from build123d import *

# Parameters (mm, degrees)
CROQUIS1_R              = 2.5
CROQUIS1_R_2            = 37.5
CROQUIS1_R_3            = 15
CROQUIS1_R_4            = 2.25
CROQUIS1_R_5            = 1.5
CROQUIS1_W              = 150
CROQUIS1_H              = 150
SALIENTE_EXTRUIR1_DEPTH = 10


with BuildPart() as part:
    # Croquis1 → Saliente-Extruir1 (new body)
    with BuildSketch(Plane.XY):
        with BuildLine():
            Line((15, 0), (485, 0))
            ThreePointArc((485, 0), (495.606601718, 4.393398282), (500, 15))
            Line((500, 15), (500, 235))
            ThreePointArc((500, 235), (495.606601718, 245.606601718), (485, 250))
            Line((485, 250), (15, 250))
            ThreePointArc((15, 250), (4.393398282, 245.606601718), (0, 235))
            Line((0, 235), (0, 15))
            ThreePointArc((0, 15), (4.393398282, 4.393398282), (15, 0))
        make_face()
        with Locations((110, 185.621778265)):
            Circle(CROQUIS1_R, mode=Mode.SUBTRACT)
        with Locations((162.5, 94.689110868)):
            Circle(CROQUIS1_R, mode=Mode.SUBTRACT)
        with Locations((57.5, 94.689110868)):
            Circle(CROQUIS1_R, mode=Mode.SUBTRACT)
        with Locations((110, 125)):
            Circle(CROQUIS1_R_2, mode=Mode.SUBTRACT)
        with Locations((230, 235)):
            Circle(CROQUIS1_R, mode=Mode.SUBTRACT)
        with Locations((270, 235)):
            Circle(CROQUIS1_R, mode=Mode.SUBTRACT)
        with Locations((189.096460098, 45)):
            Circle(CROQUIS1_R_3, mode=Mode.SUBTRACT)
        with Locations((475, 210)):
            Circle(CROQUIS1_R_4, mode=Mode.SUBTRACT)
        with Locations((305, 210)):
            Circle(CROQUIS1_R_4, mode=Mode.SUBTRACT)
        with Locations((305, 40)):
            Circle(CROQUIS1_R_4, mode=Mode.SUBTRACT)
        with Locations((475, 40)):
            Circle(CROQUIS1_R_4, mode=Mode.SUBTRACT)
        with Locations((350, 10)):
            Circle(CROQUIS1_R, mode=Mode.SUBTRACT)
        with Locations((380, 10)):
            Circle(CROQUIS1_R, mode=Mode.SUBTRACT)
        with Locations(Location((120, 10, 0), (0, 0, 180))):
            Circle(CROQUIS1_R, mode=Mode.SUBTRACT)
        with Locations(Location((150, 10, 0), (0, 0, 180))):
            Circle(CROQUIS1_R, mode=Mode.SUBTRACT)
        with Locations((240, 125)):
            Circle(CROQUIS1_R, mode=Mode.SUBTRACT)
        with Locations((260, 125)):
            Circle(CROQUIS1_R, mode=Mode.SUBTRACT)
        with Locations((250, 125)):
            Circle(CROQUIS1_R_5, mode=Mode.SUBTRACT)
        with Locations((390, 125)):
            Rectangle(CROQUIS1_W, CROQUIS1_H, mode=Mode.SUBTRACT)
    extrude(amount=SALIENTE_EXTRUIR1_DEPTH)


solid = part.part
Geometry: final body of the model. Coordinates: model frame, mm. A direction names the side the tool comes from. Round coordinates to 2 decimals unless told otherwise and drop trailing zeros. Order: outer loops, then holes, each group sorted by start corner. A loop starts at its lowest first (then second) coordinate and runs counter-clockwise, first axis right, second up. Notation, with made-up numbers: (79, -1) -> (84, -1) arc R14 cw to (84, 26) -> close; hole circle Ø11 at (7.25, 52.25). An arc over 180 degrees is marked (long way). Put each result on its own line as item: value. Start each with the question number.
Q1. Section C-C on y = 148. Return the cut outline in (x, z), and give its area (3 significant figures).
Q2. Line query: probe 1 along Y at (x, z) = (110, 3); probe 2 along X at (y, z) = (235, 6); probe 3 along Y at (x, z) = (305, 2). Output: solid intervals per line, ascending.
Q3. First-contact query: pin 1 (3 mm diameter, centred on x = 240, y = 125, fed in from +Z). Flat tip, straight axial feed; report the tip coordinate or a pass-through.
Q4. Pull-direction query (Y, two-part tool) for faces 1 (the flat face through (247, 127, 0)), 2 (the cylindrical face through (4.51, 245.72, 4.93)), 3 (the flat face through (389, 50, 5)); classes: +Y half, -Y half, draft (parallel to the pull), parting line (faces both ways), or undercut.
Q5. Section B-B on z = 7.75. Give the number of separate pieces and of enclosed holes in the cut face, and give its area (3 significant figures).
Q6. Reachability of faces 4 (the flat face through (315, 124, 5)), 5 (the flat face through (247, 0, 5)) from +Z, -Z, +X, -X, +Y, -Y: full face, straight path, thin tool, end or side. Return the list, or none.
Q7. Section A-A on x = 432. Return the cut outline in (y, z).
Ans:
1. outline: (0, 0) -> (80.38, 0) -> (80.38, 10) -> (0, 10) -> close; (139.62, 0) -> (315, 0) -> (315, 10) -> (139.62, 10) -> close; (465, 0) -> (500, 0) -> (500, 10) -> (465, 10) -> close
1. area: 2,910 mm2
2. probe 1: y = 0 to 87.5, 162.5 to 183.12, 188.12 to 250
2. probe 2: x = 0 to 227.5, 232.5 to 267.5, 272.5 to 500
2. probe 3: y = 0 to 37.75, 42.25 to 207.75, 212.25 to 250
3. pin 1: passes through
4. face 1: draft
4. face 2: +Y half
4. face 3: undercut
5. separate pieces: 1
5. enclosed holes: 19
5. area: 96,900 mm2
6. face 4: +Z, -Z
6. face 5: +Z, -Z, +X, -X, -Y
7. outline: (0, 0) -> (50, 0) -> (50, 10) -> (0, 10) -> close; (200, 0) -> (250, 0) -> (250, 10) -> (200, 10) -> close
